from build123d import *

# Parameters (mm, degrees)
EXTRUDE_2_DEPTH     = 2
SKETCH_3_R          = 1.5
CUT_EXTRUDE_1_DEPTH = 95.361008897
EXTRUDE_3_DEPTH     = 1
DRAFT_4_ANGLE       = 43
SKETCH_6_W          = 6
SKETCH_6_H          = 10
EXTRUDE_4_DEPTH     = 5
SKETCH_7_W          = 6
SKETCH_7_H          = 10
EXTRUDE_5_DEPTH     = 5
CUT_EXTRUDE_2_DEPTH = 107.596038813


with BuildPart() as part:
    # 草图1 → 凸台-拉伸2 (new body)
    with BuildSketch(Plane.XY):
        Polygon((0, 0), (0, 50), (20, 50), (20, 40), (60, 40), (60, 50), (80, 50), (80, 0), (60, 0), (60, 10), (20, 10), (20, 0), align=None)
    extrude(amount=EXTRUDE_2_DEPTH)

    # 草图3 → 切除-拉伸1 (cut, through all)
    with BuildSketch(Plane.XY.offset(2)):
        with Locations((10, 45)):
            Circle(SKETCH_3_R)
        with Locations((10, 5)):
            Circle(SKETCH_3_R)
        with Locations((70, 45)):
            Circle(SKETCH_3_R)
        with Locations((70, 5)):
            Circle(SKETCH_3_R)
    extrude(amount=-CUT_EXTRUDE_1_DEPTH, mode=Mode.SUBTRACT)

    # 草图5 → 凸台-拉伸3 (add)
    with BuildSketch(Plane.XY.offset(2)):
        with BuildLine():
            Line((0, 50), (6, 50))
            Line((6, 50), (6, 45))
            ThreePointArc((6, 45), (10, 41), (14, 45))
            Line((14, 45), (14, 50))
            Line((14, 50), (20, 50))
            Line((20, 50), (20, 40))
            Line((20, 40), (60, 40))
            Line((60, 40), (60, 50))
            Line((60, 50), (66, 50))
            Line((66, 50), (66, 45))
            ThreePointArc((66, 45), (70, 41), (74, 45))
            Line((74, 45), (74, 50))
            Line((74, 50), (80, 50))
            Line((80, 50), (80, 0))
            Line((80, 0), (74, 0))
            Line((74, 0), (74, 5))
            ThreePointArc((74, 5), (70, 9), (66, 5))
            Line((66, 5), (66, 0))
            Line((66, 0), (60, 0))
            Line((60, 0), (60, 10))
            Line((60, 10), (20, 10))
            Line((20, 10), (20, 0))
            Line((20, 0), (14, 0))
            Line((14, 0), (14, 5))
            ThreePointArc((14, 5), (10, 9), (6, 5))
            Line((6, 5), (6, 0))
            Line((6, 0), (0, 0))
            Line((0, 0), (0, 50))
        make_face()
    extrude(amount=EXTRUDE_3_DEPTH)

    # 拔模4
    draft_4_faces = [part.faces().sort_by_distance(p)[0] for p in [
        (40, 25, 3),
    ]]
    draft(draft_4_faces, Plane(origin=(20, 0, 2), x_dir=(-1, 0, 0), z_dir=(0, -1, 0)), DRAFT_4_ANGLE)

    # 草图6 → 凸台-拉伸4 (add)
    with BuildSketch(Plane(origin=(0, -1.496346075, 1.604634711), x_dir=(1, 0, 0), z_dir=(0, -0.6819983600624997, 0.7313537016191695))):
        with Locations((3, 7.04599508)):
            Rectangle(SKETCH_6_W, SKETCH_6_H)
    extrude(amount=EXTRUDE_4_DEPTH)

    # 草图7 → 凸台-拉伸5 (add)
    with BuildSketch(Plane(origin=(0, -1.496346075, 1.604634711), x_dir=(1, 0, 0), z_dir=(0, -0.6819983600624997, 0.7313537016191695))):
        with Locations((77, 7.04599508)):
            Rectangle(SKETCH_7_W, SKETCH_7_H)
    extrude(amount=EXTRUDE_5_DEPTH)

    # 草图8 → 切除-拉伸2 (cut, through all)
    with BuildSketch(Plane(origin=(80, 0, 0), x_dir=(0, 0, -1), z_dir=(1, 0, 0))):
        Polygon((-3, 0), (-9.836637305, 0), (-6.656768508, -3.4099918), align=None)
    extrude(amount=-CUT_EXTRUDE_2_DEPTH, mode=Mode.SUBTRACT)


solid = part.part
Design review of the part built by this model. Coordinates are the model's own, in mm. A direction names the side the tool comes from. Round coordinates to 2 decimals unless told otherwise and drop trailing zeros. Write each loop counter-clockwise with the first axis right and the second up, starting at its lowest first coordinate (ties: lowest second). Pieces come first, ordered by that corner, then holes. Notation, with made-up numbers: (58.25, 49.25) -> (107.25, 49.25) arc R18 cw to (107.25, 57.25) -> close; hole circle Ø4 at (45.25, 64.5). An arc over 180 degrees is marked (long way). One line per question, with ' | ' between items.
(1) Take a section at D-D, the plane x = 34.5. State the section outline as (y, z) points.
Result sheet:
outline: (10, 0) -> (40, 0) -> (40, 40.3) -> (10, 12.33) -> close
(2) Machinability: for faces 1 (the flat face through (69.17, 3.56, 2)), 2 (the flat face through (2.958, 5.632, 11.623)), 3 (the cylindrical face through (8.5, 5.07, 1.01)), 4 (the flat face through (40, 10, 6)), 5 (the flat face through (74, 47, 25)), which of the approach directions +Z, -Z, +X, -X, +Y, -Y give a long, thin tool a straight path to every point of the face, cutting with its end or side? Answer none if there is none.
Result sheet:
face 1: +Z, -Y | face 2: +Z, +X, -X | face 3: +Z, -Z | face 4: +Z, -Z, -Y | face 5: +Z, +Y
(3) Take a section at B-B, the plane x = 70. State the section outline as (y, z) points, and give its area (3 significant figures).
Result sheet:
outline: (0, 0) -> (3.5, 0) -> (3.5, 2) -> (0, 2) -> close; (6.5, 0) -> (43.5, 0) -> (43.5, 2) -> (41, 2) -> (41, 41.23) -> (9, 11.39) -> (9, 2) -> (6.5, 2) -> close; (46.5, 0) -> (50, 0) -> (50, 2) -> (46.5, 2) -> close | area: 866 mm2
(4) Insertion check: P1, Ø2.5, axis at x = 10.5, y = 47, coming from the +Z side; P2, Ø3, axis at x = 52.5, z = 8, coming from the -Y side; P3, Ø8, axis at x = 10.5, y = 39.5, coming from the +Z side. Each pin has a flat end and moves straight along its axis. Give the tip position at first contact, or say it passes through.
Result sheet:
P1: z = 2 | P2: y = 10 | P3: z = 42.64
(5) Wall thickness on line 1 (X direction, y = 47, z = 14.5); line 2 (Y direction, x = 70, z = 1.3); line 3 (Y direction, x = 44, z = 11.5): over which ranges is each line inside the solid? List them lowest first. Write a range as [from, to].
Result sheet:
line 1: [0, 6], [14, 20], [60, 66], [74, 80] | line 2: [0, 3.5], [6.5, 43.5], [46.5, 50] | line 3: [10, 40]
(6) Take a section at A-A, the plane y = 42.5. State the section outline as (x, z) points, and give its area (3 significant figures).
Result sheet:
outline: (0, 0) -> (20, 0) -> (20, 42.63) -> (13.12, 42.63) -> (13.12, 2) -> (6.88, 2) -> (6.88, 42.63) -> (0, 42.63) -> close; (60, 0) -> (80, 0) -> (80, 42.63) -> (73.12, 42.63) -> (73.12, 2) -> (66.88, 2) -> (66.88, 42.63) -> (60, 42.63) -> close | area: 1,200 mm2
(7) Take a section at C-C, the plane z = 39. State the section outline as (x, y) points.
Result sheet:
outline: (0, 38.61) -> (80, 38.61) -> (80, 50) -> (74, 50) -> (74, 45) arc R4 cw to (66, 45) -> (66, 50) -> (60, 50) -> (60, 40) -> (20, 40) -> (20, 50) -> (14, 50) -> (14, 45) arc R4 cw to (6, 45) -> (6, 50) -> (0, 50) -> close
(8) Draft analysis for pull direction X (two halves, no side actions). For faces 6 (the flat face through (6, 48, 25)), 7 (the flat face through (75, 0, 4)), state which applies: released by +X, released by -X, zero draft, split by the parting line, or undercut.
Result sheet:
face 6: undercut | face 7: zero draft
